Could you check a few things on this model? Use its own coordinates, in mm. Round coordinates to 2 decimals unless told otherwise and drop trailing zeros. Write each loop counter-clockwise with the first axis right and the second up, starting at its lowest first coordinate (ties: lowest second). Pieces come first, ordered by that corner, then holes. Notation, with made-up numbers: (56, -1) - (106, -1) arc R22 ccw to (106, 36) - close; hole circle Ø10 at (5.25, -3). An arc over 180 degrees is marked (long way). Put each result on its own line as item: value.
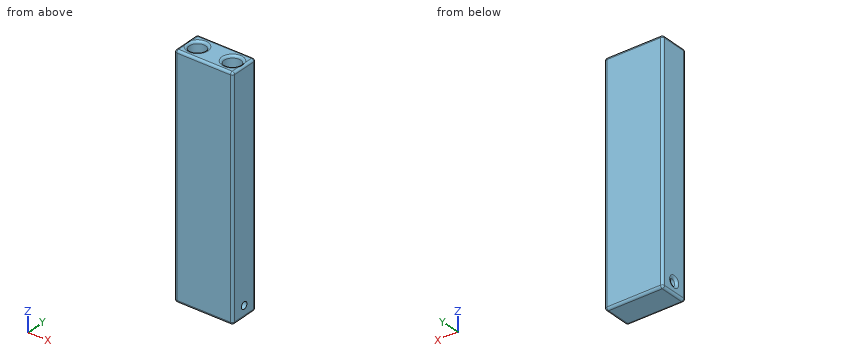
from build123d import *

# Parameters (mm, degrees)
F0_W         = 25
F0_H         = 100
F1_DEPTH     = 12.5
F2_R         = 1.5
F3_DEPTH     = 27.19003
F4_R         = 3.5
F5_DEPTH     = 10
F6_T1_DEPTH  = 10.5
F6_T3_DEPTH  = 23
F6_T5_DEPTH  = 98
F6_S9_W      = 1
F6_S9_H      = 1
F6_T10_DEPTH = 1
F6_S15_W     = 1
F6_S15_H     = 1
F6_T16_DEPTH = 1
F6_S21_W     = 1
F6_S21_H     = 1
F6_T22_DEPTH = 1
F6_S27_W     = 1
F6_S27_H     = 1
F6_T28_DEPTH = 1
F6_S33_W     = 1
F6_S33_H     = 1
F6_T34_DEPTH = 1
F6_S39_W     = 1
F6_S39_H     = 1
F6_T40_DEPTH = 1
F6_S45_W     = 1
F6_S45_H     = 1
F6_T46_DEPTH = 1
F6_S51_W     = 1
F6_S51_H     = 1
F6_T52_DEPTH = 1


# Not quite as in the source:
# - a fillet or chamfer that OpenCascade refuses, or shapes differently, is made with other operations: its cross-section is extruded or revolved along the edge and cut away or added


with BuildPart() as f1:
    # F0 (on Front) → F1 (new body)
    with BuildSketch(Plane.XZ):
        with Locations((-13.6877183104, 5.2395616682)):
            Rectangle(F0_W, F0_H)
    extrude(amount=F1_DEPTH)

    # F2 (on Right) → F3 (cut)
    with BuildSketch(Plane.YZ):
        with Locations((-6.25, -39.7604383318)):
            Circle(F2_R)
    extrude(amount=-F3_DEPTH, mode=Mode.SUBTRACT)

    # F4 (on face) → F5 (cut)
    with BuildSketch(Plane.XY.offset(55.2395616682)):
        with Locations((-6.1877183104, -6.25)):
            Circle(F4_R)
        with Locations((-21.1877183104, -6.25)):
            Circle(F4_R)
    extrude(amount=-F5_DEPTH, mode=Mode.SUBTRACT)

    # F6: fillet of radius 1 on 15 edges, made by hand

    # F6_s2 → F6_t1 (cut)
    with BuildSketch(Plane.XZ.offset(1)):
        with BuildLine():
            ThreePointArc((-25.1877183104, 55.2395616682), (-25.8948250916, 54.9466684494), (-26.1877183104, 54.2395616682))
            Line((-26.1877183104, 54.2395616682), (-26.1877183104, 55.2395616682))
            Line((-26.1877183104, 55.2395616682), (-25.1877183104, 55.2395616682))
        make_face()
        with BuildLine():
            ThreePointArc((-2.1877183104, 55.2395616682), (-1.4806115292, 54.9466684494), (-1.1877183104, 54.2395616682))
            Line((-1.1877183104, 54.2395616682), (-1.1877183104, 55.2395616682))
            Line((-1.1877183104, 55.2395616682), (-2.1877183104, 55.2395616682))
        make_face()
        with BuildLine():
            ThreePointArc((-26.1877183104, -43.7604383318), (-25.8948250916, -44.467545113), (-25.1877183104, -44.7604383318))
            Line((-25.1877183104, -44.7604383318), (-26.1877183104, -44.7604383318))
            Line((-26.1877183104, -44.7604383318), (-26.1877183104, -43.7604383318))
        make_face()
        with BuildLine():
            ThreePointArc((-1.1877183104, -43.7604383318), (-1.4806115292, -44.467545113), (-2.1877183104, -44.7604383318))
            Line((-2.1877183104, -44.7604383318), (-1.1877183104, -44.7604383318))
            Line((-1.1877183104, -44.7604383318), (-1.1877183104, -43.7604383318))
        make_face()
    extrude(amount=F6_T1_DEPTH, mode=Mode.SUBTRACT)

    # F6_s4 → F6_t3 (cut)
    with BuildSketch(Plane.YZ.offset(-25.1877183104)):
        with BuildLine():
            ThreePointArc((-11.5, 55.2395616682), (-12.2071067812, 54.9466684494), (-12.5, 54.2395616682))
            Line((-12.5, 54.2395616682), (-12.5, 55.2395616682))
            Line((-12.5, 55.2395616682), (-11.5, 55.2395616682))
        make_face()
        with BuildLine():
            ThreePointArc((-1, 55.2395616682), (-0.2928932188, 54.9466684494), (0, 54.2395616682))
            Line((0, 54.2395616682), (0, 55.2395616682))
            Line((0, 55.2395616682), (-1, 55.2395616682))
        make_face()
        with BuildLine():
            ThreePointArc((0, -43.7604383318), (-0.2928932188, -44.467545113), (-1, -44.7604383318))
            Line((-1, -44.7604383318), (0, -44.7604383318))
            Line((0, -44.7604383318), (0, -43.7604383318))
        make_face()
        with BuildLine():
            ThreePointArc((-12.5, -43.7604383318), (-12.2071067812, -44.467545113), (-11.5, -44.7604383318))
            Line((-11.5, -44.7604383318), (-12.5, -44.7604383318))
            Line((-12.5, -44.7604383318), (-12.5, -43.7604383318))
        make_face()
    extrude(amount=F6_T3_DEPTH, mode=Mode.SUBTRACT)

    # F6_s6 → F6_t5 (cut)
    with BuildSketch(Plane.XY.offset(-43.7604383318)):
        with BuildLine():
            ThreePointArc((-25.1877183104, 0), (-25.8948250916, -0.2928932188), (-26.1877183104, -1))
            Line((-26.1877183104, -1), (-26.1877183104, 0))
            Line((-26.1877183104, 0), (-25.1877183104, 0))
        make_face()
        with BuildLine():
            ThreePointArc((-1.1877183104, -1), (-1.4806115292, -0.2928932188), (-2.1877183104, 0))
            Line((-2.1877183104, 0), (-1.1877183104, 0))
            Line((-1.1877183104, 0), (-1.1877183104, -1))
        make_face()
        with BuildLine():
            ThreePointArc((-25.1877183104, -12.5), (-25.8948250916, -12.2071067812), (-26.1877183104, -11.5))
            Line((-26.1877183104, -11.5), (-26.1877183104, -12.5))
            Line((-26.1877183104, -12.5), (-25.1877183104, -12.5))
        make_face()
        with BuildLine():
            ThreePointArc((-1.1877183104, -11.5), (-1.4806115292, -12.2071067812), (-2.1877183104, -12.5))
            Line((-2.1877183104, -12.5), (-1.1877183104, -12.5))
            Line((-1.1877183104, -12.5), (-1.1877183104, -11.5))
        make_face()
    extrude(amount=F6_T5_DEPTH, mode=Mode.SUBTRACT)


with BuildPart() as f6_tool8:
    # F6_s9 → F6_t10 (new body)
    with BuildSketch(Plane.XY.offset(54.2395616682)):
        with Locations((-25.6877183104, -0.5)):
            Rectangle(F6_S9_W, F6_S9_H)
    extrude(amount=F6_T10_DEPTH)

    # F6_s11 → F6_t12 (revolve, cut)
    with BuildSketch(Plane(origin=(-25.1877183104, -1, 54.2395616682), x_dir=(0.7071067812, -0.7071067812, 0), z_dir=(-0.7071067812, -0.7071067812, 0))):
        with BuildLine():
            ThreePointArc((0, -1), (1, 0), (0, 1))
            Line((0, 1), (0, -1))
        make_face()
    revolve(axis=Axis((-25.1877183104, -1, 54.2395616682), (0, 0, 1)), mode=Mode.SUBTRACT)


with BuildPart() as f1_1:
    add(f1.part)

    # F6_t7: cut F6_tool8
    add(f6_tool8.part, mode=Mode.SUBTRACT)


with BuildPart() as f6_tool14:
    # F6_s15 → F6_t16 (new body)
    with BuildSketch(Plane.XY.offset(54.2395616682)):
        with Locations((-25.6877183104, -12)):
            Rectangle(F6_S15_W, F6_S15_H)
    extrude(amount=F6_T16_DEPTH)

    # F6_s17 → F6_t18 (revolve, cut)
    with BuildSketch(Plane(origin=(-25.1877183104, -11.5, 54.2395616682), x_dir=(0.7071067812, 0.7071067812, 0), z_dir=(0.7071067812, -0.7071067812, 0))):
        with BuildLine():
            ThreePointArc((0, -1), (1, 0), (0, 1))
            Line((0, 1), (0, -1))
        make_face()
    revolve(axis=Axis((-25.1877183104, -11.5, 54.2395616682), (0, 0, 1)), mode=Mode.SUBTRACT)


with BuildPart() as f1_2:
    add(f1_1.part)

    # F6_t13: cut F6_tool14
    add(f6_tool14.part, mode=Mode.SUBTRACT)


with BuildPart() as f6_tool20:
    # F6_s21 → F6_t22 (new body)
    with BuildSketch(Plane.XY.offset(54.2395616682)):
        with Locations((-1.6877183104, -12)):
            Rectangle(F6_S21_W, F6_S21_H)
    extrude(amount=F6_T22_DEPTH)

    # F6_s23 → F6_t24 (revolve, cut)
    with BuildSketch(Plane(origin=(-2.1877183104, -11.5, 54.2395616682), x_dir=(-0.7071067812, 0.7071067812, 0), z_dir=(0.7071067812, 0.7071067812, 0))):
        with BuildLine():
            ThreePointArc((0, -1), (1, 0), (0, 1))
            Line((0, 1), (0, -1))
        make_face()
    revolve(axis=Axis((-2.1877183104, -11.5, 54.2395616682), (0, 0, 1)), mode=Mode.SUBTRACT)


with BuildPart() as f1_3:
    add(f1_2.part)

    # F6_t19: cut F6_tool20
    add(f6_tool20.part, mode=Mode.SUBTRACT)


with BuildPart() as f6_tool26:
    # F6_s27 → F6_t28 (new body)
    with BuildSketch(Plane.XY.offset(54.2395616682)):
        with Locations((-1.6877183104, -0.5)):
            Rectangle(F6_S27_W, F6_S27_H)
    extrude(amount=F6_T28_DEPTH)

    # F6_s29 → F6_t30 (revolve, cut)
    with BuildSketch(Plane(origin=(-2.1877183104, -1, 54.2395616682), x_dir=(-0.7071067812, -0.7071067812, 0), z_dir=(-0.7071067812, 0.7071067812, 0))):
        with BuildLine():
            ThreePointArc((0, -1), (1, 0), (0, 1))
            Line((0, 1), (0, -1))
        make_face()
    revolve(axis=Axis((-2.1877183104, -1, 54.2395616682), (0, 0, 1)), mode=Mode.SUBTRACT)


with BuildPart() as f1_4:
    add(f1_3.part)

    # F6_t25: cut F6_tool26
    add(f6_tool26.part, mode=Mode.SUBTRACT)


with BuildPart() as f6_tool32:
    # F6_s33 → F6_t34 (new body)
    with BuildSketch(Plane.XZ.offset(1)):
        with Locations((-25.6877183104, -44.2604383318)):
            Rectangle(F6_S33_W, F6_S33_H)
    extrude(amount=-F6_T34_DEPTH)

    # F6_s35 → F6_t36 (revolve, cut)
    with BuildSketch(Plane(origin=(-25.1877183104, -1, -43.7604383318), x_dir=(0.7071067812, 0, 0.7071067812), z_dir=(-0.7071067812, 0, 0.7071067812))):
        with BuildLine():
            ThreePointArc((0, -1), (1, 0), (0, 1))
            Line((0, 1), (0, -1))
        make_face()
    revolve(axis=Axis((-25.1877183104, -1, -43.7604383318), (0, 1, 0)), mode=Mode.SUBTRACT)


with BuildPart() as f1_5:
    add(f1_4.part)

    # F6_t31: cut F6_tool32
    add(f6_tool32.part, mode=Mode.SUBTRACT)


with BuildPart() as f6_tool38:
    # F6_s39 → F6_t40 (new body)
    with BuildSketch(Plane.YZ.offset(-2.1877183104)):
        with Locations((-0.5, -44.2604383318)):
            Rectangle(F6_S39_W, F6_S39_H)
    extrude(amount=F6_T40_DEPTH)

    # F6_s41 → F6_t42 (revolve, cut)
    with BuildSketch(Plane(origin=(-2.1877183104, -1, -43.7604383318), x_dir=(0, -0.7071067812, 0.7071067812), z_dir=(0, 0.7071067812, 0.7071067812))):
        with BuildLine():
            ThreePointArc((0, -1), (1, 0), (0, 1))
            Line((0, 1), (0, -1))
        make_face()
    revolve(axis=Axis((-2.1877183104, -1, -43.7604383318), (1, 0, 0)), mode=Mode.SUBTRACT)


with BuildPart() as f1_6:
    add(f1_5.part)

    # F6_t37: cut F6_tool38
    add(f6_tool38.part, mode=Mode.SUBTRACT)


with BuildPart() as f6_tool44:
    # F6_s45 → F6_t46 (new body)
    with BuildSketch(Plane.XZ.offset(11.5)):
        with Locations((-25.6877183104, -44.2604383318)):
            Rectangle(F6_S45_W, F6_S45_H)
    extrude(amount=F6_T46_DEPTH)

    # F6_s47 → F6_t48 (revolve, cut)
    with BuildSketch(Plane(origin=(-25.1877183104, -11.5, -43.7604383318), x_dir=(0.7071067812, 0, 0.7071067812), z_dir=(0.7071067812, 0, -0.7071067812))):
        with BuildLine():
            ThreePointArc((0, -1), (1, 0), (0, 1))
            Line((0, 1), (0, -1))
        make_face()
    revolve(axis=Axis((-25.1877183104, -11.5, -43.7604383318), (0, -1, 0)), mode=Mode.SUBTRACT)


with BuildPart() as f1_7:
    add(f1_6.part)

    # F6_t43: cut F6_tool44
    add(f6_tool44.part, mode=Mode.SUBTRACT)


with BuildPart() as f6_tool50:
    # F6_s51 → F6_t52 (new body)
    with BuildSketch(Plane.YZ.offset(-2.1877183104)):
        with Locations((-12, -44.2604383318)):
            Rectangle(F6_S51_W, F6_S51_H)
    extrude(amount=F6_T52_DEPTH)

    # F6_s53 → F6_t54 (revolve, cut)
    with BuildSketch(Plane(origin=(-2.1877183104, -11.5, -43.7604383318), x_dir=(0, 0.7071067812, 0.7071067812), z_dir=(0, 0.7071067812, -0.7071067812))):
        with BuildLine():
            ThreePointArc((0, -1), (1, 0), (0, 1))
            Line((0, 1), (0, -1))
        make_face()
    revolve(axis=Axis((-2.1877183104, -11.5, -43.7604383318), (1, 0, 0)), mode=Mode.SUBTRACT)


with BuildPart() as f1_8:
    add(f1_7.part)

    # F6_t49: cut F6_tool50
    add(f6_tool50.part, mode=Mode.SUBTRACT)

    # F6_s55 → F6_t56 (revolve, cut)
    with BuildSketch(Plane.XY.offset(-39.7604383318)):
        with BuildLine():
            ThreePointArc((-26.1877183104, -3.75), (-25.8948250916, -4.4571067812), (-25.1877183104, -4.75))
            Line((-25.1877183104, -4.75), (-26.1877183104, -4.75))
            Line((-26.1877183104, -4.75), (-26.1877183104, -3.75))
        make_face()
    revolve(axis=Axis((-26.1877183104, -6.25, -39.7604383318), (1, 0, 0)), mode=Mode.SUBTRACT)

    # F6_s57 → F6_t58 (revolve, cut)
    with BuildSketch(Plane.XZ.offset(6.25)):
        with BuildLine():
            ThreePointArc((-16.6877183104, 55.2395616682), (-17.3948250916, 54.9466684494), (-17.6877183104, 54.2395616682))
            Line((-17.6877183104, 54.2395616682), (-17.6877183104, 55.2395616682))
            Line((-17.6877183104, 55.2395616682), (-16.6877183104, 55.2395616682))
        make_face()
    revolve(axis=Axis((-21.1877183104, -6.25, 55.2395616682), (0, 0, 1)), mode=Mode.SUBTRACT)

    # F6_s59 → F6_t60 (revolve, cut)
    with BuildSketch(Plane.XZ.offset(6.25)):
        with BuildLine():
            ThreePointArc((-1.6877183104, 55.2395616682), (-2.3948250916, 54.9466684494), (-2.6877183104, 54.2395616682))
            Line((-2.6877183104, 54.2395616682), (-2.6877183104, 55.2395616682))
            Line((-2.6877183104, 55.2395616682), (-1.6877183104, 55.2395616682))
        make_face()
    revolve(axis=Axis((-6.1877183104, -6.25, 55.2395616682), (0, 0, 1)), mode=Mode.SUBTRACT)


solid = f1_8.part
(1) I'm going to push flat-ended pins straight in: pin 1 (7.5 mm diameter, centred on x = -8, y = -7.5, fed in from +Z); pin 2 (2 mm diameter, centred on x = -22, y = -4.5, fed in from +Z). Where does each tip first touch, or does it pass through?
Values found:
pin 1: stops at z = 55.24
pin 2: stops at z = 45.24
(2) Please list where these lines run through material, in increasing order: probe 1 along Z at (x, y) = (-12.25, -6.25); probe 2 along Z at (x, y) = (-7.5, -6.25); probe 3 along Z at (x, y) = (-21, -3). Write a range as from..to.
Values found:
probe 1: z = -44.76..-41.26, -38.26..55.24
probe 2: z = -44.76..-41.26, -38.26..45.24
probe 3: z = -44.76..45.24
(3) Imagine slicing it at A-A, the plane y = -6.25. List the corners of the cut face in (x, z) for me, then the cut area to 3 significant figures.
Values found:
outline: (-26.19, -43.76) arc R1 ccw to (-25.19, -44.76) - (-2.19, -44.76) arc R1 ccw to (-1.19, -43.76) - (-1.19, -41.26) - (-25.19, -41.26) arc R1 ccw to (-26.19, -42.26) - close; (-26.19, -37.26) arc R1 ccw to (-25.19, -38.26) - (-1.19, -38.26) - (-1.19, 54.24) arc R1 ccw to (-1.94, 55.21) arc R1 ccw to (-2.69, 54.24) - (-2.69, 45.24) - (-9.69, 45.24) - (-9.69, 54.24) arc R1 ccw to (-10.69, 55.24) - (-16.69, 55.24) arc R1 ccw to (-17.69, 54.24) - (-17.69, 45.24) - (-24.69, 45.24) - (-24.69, 54.24) arc R1 ccw to (-25.44, 55.21) arc R1 ccw to (-26.19, 54.24) - close
area: 2,280 mm^2
